Part model, mm, in its own coordinate system. Face numbers are marked on the shaded views. A direction names the side the tool comes from. Give positions to 0.01 mm unless a question says otherwise; leave off trailing zeros. Write each loop counter-clockwise with the first axis right and the second up, starting at its lowest first coordinate (ties: lowest second). Pieces come first, ordered by that corner, then holes.
from build123d import *

# Parameters (mm, degrees)
F0_R     = 4.365625
F1_DEPTH = 14.2875
F2_R     = 3.175
F3_DEPTH = 38.1
F4_R     = 3.175
F5_DEPTH = 12.7


with BuildPart() as f1:
    # F0 (on Front) → F1 (new body)
    with BuildSketch(Plane.XZ):
        Circle(F0_R)
    extrude(amount=F1_DEPTH)

    # F2 (on face) → F3 (join)
    with BuildSketch(Plane.XZ.offset(14.2875)):
        Circle(F2_R)
    extrude(amount=F3_DEPTH)

    # F4 (on face) → F5 (cut)
    with BuildSketch(Plane.XZ.offset(52.3875)):
        Circle(F4_R)
        Polygon((0, -2.749631), (-2.38125, -1.374815), (-2.38125, 1.374815), (0, 2.749631), (2.38125, 1.374815), (2.38125, -1.374815), align=None, mode=Mode.SUBTRACT)
    extrude(amount=-F5_DEPTH, mode=Mode.SUBTRACT)


solid = f1.part
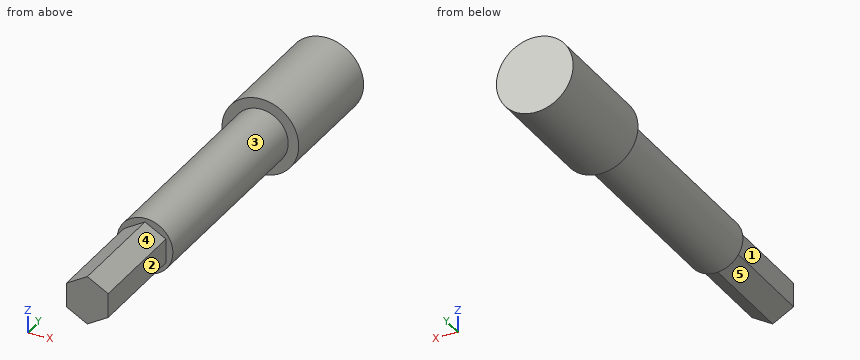
1) Saw through at C-C (y = -40.5). Write the cut outline in (x, z), and give its area (3 significant figures).
Check result:
outline: (-2.38, -1.37) - (0, -2.75) - (2.38, -1.37) - (2.38, 1.37) - (0, 2.75) - (-2.38, 1.37) - close
area: 19.6 mm2
2) Saw through at D-D (y = -34). Write the cut outline in (x, z) (3 decimals).
Check result:
outline: circle Ø6.35 at (0, 0)
3) Saw through at B-B (x = -1.25). Write the cut outline in (y, z), and give its area (3 significant figures).
Check result:
outline: (-52.39, -2.03) - (-39.69, -2.03) - (-39.69, -2.92) - (-14.29, -2.92) - (-14.29, -4.18) - (0, -4.18) - (0, 4.18) - (-14.29, 4.18) - (-14.29, 2.92) - (-39.69, 2.92) - (-39.69, 2.03) - (-52.39, 2.03) - close
area: 319 mm2
4) Flat gauge pins, fed straight in: P1, Ø1.5, axis at y = -9.5, z = 1, coming from the +X side; P2, Ø0.8, axis at y = -44.5, z = -0.5, coming from the +X side; P3, Ø2, axis at x = 1, y = -25, coming from the -Z side (3 decimals). Where does each tip first touch, or does it go through?
Check result:
P1: stops at x = 4.36
P2: stops at x = 2.38
P3: stops at z = -3.175
5) Saw through at A-A (z = 0). Write the cut outline in (x, y) (1 decimal), and give its area (3 significant figures).
Check result:
outline: (-4.4, -14.3) - (-3.2, -14.3) - (-3.2, -39.7) - (-2.4, -39.7) - (-2.4, -52.4) - (2.4, -52.4) - (2.4, -39.7) - (3.2, -39.7) - (3.2, -14.3) - (4.4, -14.3) - (4.4, 0) - (-4.4, 0) - close
area: 347 mm2
6) 3-axis set-ups, long thin cutter, end or side, ignore diameter. For the marked faces 1, 2, 3, 4 and 5: which of +Z, -Z, +X, -X, +Y, -Y reach the whole face in a straight line?
Check result:
face 1: +Z, -Z, -X, -Y
face 2: +Z, -Z, +X, -Y
face 3: -Y
face 4: +Z, +X, -Y
face 5: -Z, -X, -Y
7) Drill centre lines: L1, parallel to Z at x = 0, y = -25.5 (3 decimals); L2, parallel to Y at x = 2.5, z = -2.5; L3, parallel to Y at x = -1.5, z = -2. Where is each one in solid material? Low to high.
Check result:
L1: z = -3.175 to 3.175
L2: y = -14.29 to 0
L3: y = -39.69 to 0
